For this review, take the finished solid that the model builds, in its own axes (mm). A direction names the side the tool comes from. Give positions to 0.01 mm unless a question says otherwise; leave off trailing zeros. Order: outer loops, then holes, each group sorted by start corner. A loop starts at its lowest first (then second) coordinate and runs counter-clockwise, first axis right, second up. Notation, with made-up numbers: (7, 69.5) - (54, 69.5) arc R18 cw to (54, 83.5) - close; hole circle Ø6 at (13, -37). An arc over 180 degrees is marked (long way). Use a Markdown table: item, result. Add a question column.
1) Mouldability with a two-part tool opening along Z and no side actions: class faces 5 (the face through (0.9, 2.91, 2.86)), 6 (the face through (1.472, 4.937, 4.674)), 7 (the face through (-2.6, 4, 4.4)) as released by +Z, released by -Z, zero draft, split by the parting line, or undercut.
2) Machinability: for faces 1 (the face through (2.6, 4, 4.4)), 2 (the face through (-2.6, 4, -4.4)), 3 (the face through (5.1, 4, 0)), 4 (the face through (2.6, 4, -4.4)), which of the approach directions +Z, -Z, +X, -X, +Y, -Y give a long, thin tool a straight path to every point of the face, cutting with its end or side? Answer none if there is none.
3) We need section D-D on z = 4. Write out the cut boundary in (x, y).
4) Clearance check with flat-ended pins moving along their axes: P1, Ø1, axis at x = -2.5, y = 5, coming from the +Z side; P2, Ø1, axis at x = -0.5, z = 0.5, coming from the -Y side; P3, Ø1, axis at y = 2.5, z = 1.5, coming from the +X side. State where each tip first meets the part, or that it passes through.
5) Wall thickness on L1, parallel to Z at x = 0, y = 3.35; L2, parallel to Z at x = -1, y = 3.9; L3, parallel to Y at x = -5, z = -0.25: over which ranges is each line inside the solid? List them lowest first.
6) We need section A-A on x = 1.75. Write out the cut boundary in (y, z).
7) We need section C-C on y = 1.6. Write out the cut boundary in (x, z), then the cut area to 3 significant figures.
```python
from build123d import *

# Parameters (mm, degrees)
EXTRUDE_1_DEPTH     = 4
EXTRUDE_START       = 4
SKETCH_2_R          = 4.9
EXTRUDE_2_DEPTH     = 1.9
CUT_EXTRUDE_1_REACH = 11.531
SKETCH_3_R          = 3


with BuildPart() as part:
    # 草图1 → 凸台-拉伸1 (new body)
    with BuildSketch(Plane(origin=(0, 0, 0), x_dir=(1, 0, 0), z_dir=(0, 1, 0))):
        Polygon((5.658032638, 0), (2.829016319, 4.9), (-2.829016319, 4.9), (-5.658032638, 0), (-2.829016319, -4.9), (2.829016319, -4.9), align=None)
    extrude(amount=EXTRUDE_1_DEPTH)

    # 草图2 → 凸台-拉伸2 (add)
    with BuildSketch(Plane(origin=(0, 0, 0), x_dir=(1, 0, 0), z_dir=(0, 1, 0)).offset(EXTRUDE_START)):
        with Locations(Location((0, 0, 0), (0, 0, 270))):
            Circle(SKETCH_2_R)
    extrude(amount=EXTRUDE_2_DEPTH)

    # 草图3 → 切除-拉伸1 (cut, up to next)
    with BuildSketch(Plane(origin=(0, 0, 0), x_dir=(1, 0, 0), z_dir=(0, 1, 0)), mode=Mode.PRIVATE) as cut_extrude_1_sk1:
        with Locations(Location((0, 0, 0), (0, 0, 270))):
            Circle(SKETCH_3_R)
    cut_extrude_1_tool1 = extrude(cut_extrude_1_sk1.sketch, amount=CUT_EXTRUDE_1_REACH, mode=Mode.PRIVATE) & part.part
    add(cut_extrude_1_tool1.solids().sort_by_distance((0, 0, 0))[0], mode=Mode.SUBTRACT)


solid = part.part
```
Checked values:
| question | item | result |
|---|---|---|
| 1 | face 5 | undercut |
| 1 | face 6 | split by the parting line |
| 1 | face 7 | zero draft |
| 2 | face 1 | +Z, +X, +Y |
| 2 | face 2 | -Z, -X, +Y |
| 2 | face 3 | +X, +Y |
| 2 | face 4 | -Z, +X, +Y |
| 3 | outline | (-3.35, 0) - (3.35, 0) - (3.35, 4) - (2.83, 4) - (2.83, 5.9) - (-2.83, 5.9) - (-2.83, 4) - (-3.35, 4) - close |
| 4 | P1 | z = 4.47 |
| 4 | P2 | through |
| 4 | P3 | x = 5.08 |
| 5 | L1 | -4.9 to -3, 3 to 4.9 |
| 5 | L2 | -4.9 to -2.83, 2.83 to 4.9 |
| 5 | L3 | 0 to 4 |
| 6 | outline | (0, -4.9) - (4, -4.9) - (4, -4.58) - (5.9, -4.58) - (5.9, -2.44) - (0, -2.44) - close; (0, 2.44) - (5.9, 2.44) - (5.9, 4.58) - (4, 4.58) - (4, 4.9) - (0, 4.9) - close |
| 7 | outline | (-5.66, 0) - (-2.83, -4.9) - (2.83, -4.9) - (5.66, 0) - (2.83, 4.9) - (-2.83, 4.9) - close; hole circle Ø6 at (0, 0) |
| 7 | area | 54.9 mm² |
